Autodesk Inventor part; units mm, degrees
ref_plane "YZ Plane" through (0, 0, 0) normal (1, 0, 0) x (0, 1, 0)
ref_plane "XZ Plane" through (0, 0, 0) normal (0, 1, 0) x (-1, 0, 0)
ref_plane "XY Plane" through (0, 0, 0) normal (0, 0, 1) x (1, 0, 0)
sketch "Boceto1" plane through (0, 0, 0) normal (0, 1, 0) x (-1, 0, 0)
  line L0 (200, 200) -> (-200, 200)
  line L1 (-200, 200) -> (-200, -200)
  line L2 (-200, -200) -> (200, -200)
  line L3 (200, -200) -> (200, 200)
  point P0 (0, 0)
  dimension "d0" = 400
  dimension "L" = 400
  dimension "d2" = 200
  dimension "d3" = 200
extrude "Extrusión1" add sketch "Boceto1" along normal blind 150
sketch "Boceto3" plane through (0, 150, 0) normal (0, 1, 0) x (1, 0, 0)
  circle A0 centre (0, -121) radius 39
  line L0 (200, 200) -> (-200, 200)
  line L1 (-200, -200) -> (200, -200)
  point P0 (0, 0)
  dimension "D" = 78
  dimension "d27" = 79
extrude "Extrusión2" cut sketch "Boceto3" against normal blind 153.75
ref_plane "Plano de trabajo1" through (0, 0, 200) normal (1, 0, 0) x (0, 0, -1)
ref_plane "Plano de trabajo2" through (-200, 0, 0) normal (0, 0, 1) x (1, 0, 0)
sketch "Boceto4" plane through (0, 150, 0) normal (0, 1, 0) x (1, 0, 0)
  line L0 (-97.5, 140) -> (-97.5, -140)
  line L1 (97.5, 140) -> (97.5, -140)
  line L2 (200, 200) -> (-200, 200)
  circle A0 centre (0, -121) radius 39
  line L3 (-200, -200) -> (200, -200)
  line L4 (-97.5, -140) -> (-107.5, -140)
  line L5 (-107.5, -140) -> (-107.5, 140)
  line L6 (-107.5, 140) -> (-97.5, 140)
  line L7 (-97.5, 140) -> (-97.5, -140)
  line L8 (97.5, -140) -> (107.5, -140)
  line L9 (107.5, -140) -> (107.5, 140)
  line L10 (107.5, 140) -> (97.5, 140)
  line L11 (97.5, 140) -> (97.5, -140)
  point P0 (0, 0)
  dimension "Lriel" = 280
  dimension "d13" = 60
  dimension "d14" = 280
  dimension "d15" = 60
  dimension "d19" = 10
  dimension "d20" = 280
  dimension "d21" = 97.5
  dimension "d22" = 10
  dimension "d23" = 280
  dimension "d24" = 97.5
extrude "Extrusión3" add sketch "Boceto4" along normal blind 38 contours L0 L4 L5 L6 | L10 L9 L8 L1
sketch "Boceto5" plane through (0, 150, 0) normal (0, 1, 0) x (1, 0, 0)
  line L0 (-200, 200) -> (-200, -200)
  line L1 (-200, 200) -> (-200, 175)
  line L2 (-200, 175.482) -> (-195, 175.482)
  line L3 (-195, 175.482) -> (-195, 195.482)
  line L4 (-195, 195.482) -> (-175, 195.482)
  line L5 (-175, 195.482) -> (-175, 200)
  line L6 (200, 200) -> (-200, 200)
  line L7 (-200, 200) -> (-175, 200)
  line L8 (-200, -200) -> (-200, -175)
  line L9 (-200, -175) -> (-195, -175)
  line L10 (-195, -175) -> (-195, -195)
  line L11 (-195, -195) -> (-175, -195)
  line L12 (-175, -195) -> (-175, -200)
  line L13 (-200, -200) -> (200, -200)
  line L14 (-175, -200) -> (-200, -200)
  line L15 (200, -200) -> (200, 200)
  line L16 (200, -200) -> (200, -175)
  line L17 (200, -175) -> (195, -175)
  line L18 (195, -175) -> (195, -195)
  line L19 (195, -195) -> (175, -195)
  line L20 (175, -195) -> (175, -200)
  line L21 (200, -200) -> (175, -200)
  line L22 (200, 200) -> (200, 175)
  line L23 (200, 175) -> (195, 175)
  line L24 (195, 175) -> (195, 195)
  line L25 (195, 195) -> (175, 195)
  line L26 (175, 195) -> (175, 200)
  line L27 (200, 200) -> (175, 200)
  point P0 (0, 0)
  dimension "d28" = 25
  dimension "d29" = 5
  dimension "d30" = 20
  dimension "d31" = 20
  dimension "d32" = 25
  dimension "d33" = 5
  dimension "d34" = 20
  dimension "d35" = 20
  dimension "d36" = 25
  dimension "d37" = 5
  dimension "d38" = 20
  dimension "d39" = 20
  dimension "d40" = 25
  dimension "d41" = 5
  dimension "d42" = 20
  dimension "d43" = 20
extrude "Extrusión4" add sketch "Boceto5" along normal blind 200 contours L6 L5 L4 L3 L2 L0 | L6 L15 L23 L24 L25 L26 | L9 L10 L11 L12 L13 L0 | L15 L13 L20 L19 L18 L17
sketch "Boceto6" plane through (0, 350, 0) normal (0, 1, 0) x (1, 0, 0)
  line L0 (-200, 200) -> (-200, -200)
  line L1 (-200, -200) -> (200, -200)
  line L2 (200, -200) -> (200, 200)
  line L3 (200, 200) -> (-200, 200)
  line L4 (-200, 200) -> (-200, -200)
  point P0 (0, 0)
extrude "Extrusión5" add sketch "Boceto6" along normal blind 5
equation "\"d0\" = L"
equation "\"d14\" = Lriel"
properties part number "CajaBoya"
Work out the finished part from the listing and answer in its coordinate system (mm). A direction names the side the tool comes from. Round coordinates to 2 decimals unless told otherwise and drop trailing zeros. Write each loop counter-clockwise with the first axis right and the second up, starting at its lowest first coordinate (ties: lowest second). Pieces come first, ordered by that corner, then holes.
1) Flat-ended cylindrical pins translate along their axes: P1, Ø3, axis at x = -100.5, y = 176, coming from the -Z side; P2, Ø3, axis at x = -55, z = -62, coming from the -Y side; P3, Ø11.5, axis at y = 172, z = -63.5, coming from the +X side; P4, Ø5, axis at x = 104, y = 169, coming from the +Z side. Find the tip coordinate at first contact, or state that the pin passes through.
2) A cutting plane is placed at D-D on x = 0. Determine the outline of the cut face in (y, z).
3) Consider probe 1 along X at (y, z) = (170, -65); probe 2 along Y at (x, z) = (-6, -23); probe 3 along Z at (x, y) = (0, 79.5). Determine where each line is inside the solid, lowest interval first.
4) A cutting plane is placed at A-A on x = 156. Determine the outline of the cut face in (y, z), and give its area (3 significant figures).
5) Which of the six approach directions +Z, -Z, +X, -X, +Y, -Y give full straight-line access (tool end or side, diameter ignored) to faces 4 (the face through (17.996, 76.05, 155.6)), 5 (the face through (97.5, 169, -2)), 6 (the face through (195, 249, -185)), 7 (the face through (-107.5, 169, 2)), 8 (the face through (107.5, 169, 2))?
6) A cutting plane is placed at C-C on y = 262. Determine the outline of the cut face in (x, z).
7) Determine the mould class of faces 1 (the face through (-185, 249, -195.482)), 2 (the face through (3, 0, 3)), 3 (the face through (200, 96, 3)) for opening direction X: pulls with the +X half, pulls with the -X half, needs draft (parallel to the pull), parting line crosses it, or undercut.
8) A cutting plane is placed at B-B on z = -130. Determine the outline of the cut face in (x, y), and give its area (3 significant figures).
Entries:
1. P1: stops at z = -140
1. P2: stops at y = 0
1. P3: stops at x = 107.5
1. P4: stops at z = 140
2. outline: (0, -200) - (150, -200) - (150, 82) - (0, 82) - close; (0, 160) - (150, 160) - (150, 200) - (0, 200) - close; (350, -200) - (355, -200) - (355, 200) - (350, 200) - close
3. probe 1: x = -107.5 to -97.5, 97.5 to 107.5
3. probe 2: y = 0 to 150, 350 to 355
3. probe 3: z = -200 to 82, 160 to 200
4. outline: (0, -200) - (150, -200) - (150, 200) - (0, 200) - close; (350, -200) - (355, -200) - (355, 200) - (350, 200) - close
4. area: 62,000 mm2
5. face 4: -Y
5. face 5: +Z, -Z
5. face 6: none
5. face 7: +Z, -Z, -X
5. face 8: +Z, -Z, +X
6. outline: (-200, -200) - (-175, -200) - (-175, -195.48) - (-195, -195.48) - (-195, -175.48) - (-200, -175.48) - close; (-200, 175) - (-195, 175) - (-195, 195) - (-175, 195) - (-175, 200) - (-200, 200) - close; (175, -200) - (200, -200) - (200, -175) - (195, -175) - (195, -195) - (175, -195) - close; (175, 195) - (195, 195) - (195, 175) - (200, 175) - (200, 200) - (175, 200) - close
7. face 1: undercut
7. face 2: needs draft
7. face 3: pulls with the +X half
8. outline: (-200, 0) - (200, 0) - (200, 150) - (107.5, 150) - (107.5, 188) - (97.5, 188) - (97.5, 150) - (-97.5, 150) - (-97.5, 188) - (-107.5, 188) - (-107.5, 150) - (-200, 150) - close; (-200, 350) - (200, 350) - (200, 355) - (-200, 355) - close
8. area: 62,800 mm2
